```python
from build123d import *

# Parameters (mm, degrees)
F1_DEPTH = 10


with BuildPart() as f1:
    # F0 (on Front) → F1 (new body)
    with BuildSketch(Plane.XZ):
        with BuildLine():
            ThreePointArc((-34.337593, 36.377659), (-39.128216, 31.167084), (-43.135461, 25.332518))
            ThreePointArc((-43.135461, 25.332518), (-45.923647, 19.834894), (-48.014505, 14.036086))
            ThreePointArc((-48.014505, 14.036086), (-49.519107, 7.089604), (-50.024038, 0))
            ThreePointArc((-50.024038, 0), (-50.020463, -0.5981), (-50.009736, -1.196115))
            ThreePointArc((-50.009736, -1.196115), (-49.341893, -8.232983), (-47.688879, -15.105469))
            ThreePointArc((-47.688879, -15.105469), (-46.725007, -17.865557), (-45.601542, -20.564625))
            ThreePointArc((-45.601542, -20.564625), (-42.251133, -26.781453), (-38.058637, -32.464513))
            ThreePointArc((-38.058637, -32.464513), (-34.360112, -36.35639), (-30.265785, -39.82947))
            ThreePointArc((-30.265785, -39.82947), (-24.362413, -43.6907), (-17.974608, -46.683165))
            ThreePointArc((-17.974608, -46.683165), (-12.820651, -48.353235), (-7.516311, -49.456137))
            ThreePointArc((-7.516311, -49.456137), (-0.470356, -50.021827), (6.584991, -49.588732))
            ThreePointArc((6.584991, -49.588732), (11.499056, -48.684455), (16.298397, -47.294467))
            ThreePointArc((16.298397, -47.294467), (22.803128, -44.524395), (28.852373, -40.864961))
            ThreePointArc((28.852373, -40.864961), (32.363977, -38.144166), (35.620358, -35.122564))
            ThreePointArc((35.620358, -35.122564), (40.222649, -29.741266), (44.019019, -23.764057))
            ThreePointArc((44.019019, -23.764057), (45.828281, -20.054253), (47.32555, -16.207922))
            ThreePointArc((47.32555, -16.207922), (49.138207, -9.372354), (49.968834, -2.349478))
            ThreePointArc((49.968834, -2.349478), (50.010235, -1.175063), (50.024038, 0))
            ThreePointArc((50.024038, 0), (49.77315, 5.003793), (49.023002, 9.957394))
            ThreePointArc((49.023002, 9.957394), (47.119504, 16.797522), (44.266789, 23.299265))
            ThreePointArc((44.266789, 23.299265), (41.258147, 28.287272), (37.690051, 32.891708))
            ThreePointArc((37.690051, 32.891708), (32.67536, 37.877768), (27.007686, 42.10688))
            ThreePointArc((27.007686, 42.10688), (20.698662, 45.540858), (13.962862, 48.03585))
            ThreePointArc((13.962862, 48.03585), (7.051851, 49.524497), (0, 50.024038))
            ThreePointArc((0, 50.024038), (-7.417006, 49.471127), (-14.670053, 47.824616))
            ThreePointArc((-14.670053, 47.824616), (-21.285063, 45.269753), (-27.47235, 41.805196))
            ThreePointArc((-27.47235, 41.805196), (-31.023891, 39.241847), (-34.337593, 36.377659))
        make_face()
        with BuildLine():
            Line((-39.461789, 39.611867), (-43.135461, 25.332518))
            ThreePointArc((-43.135461, 25.332518), (-39.128216, 31.167084), (-34.337593, 36.377659))
            Line((-34.337593, 36.377659), (-39.461789, 39.611867))
        make_face()
        with BuildLine():
            ThreePointArc((-50.024038, 0), (-49.519107, 7.089604), (-48.014505, 14.036086))
            Line((-48.014505, 14.036086), (-54.538898, 14.036086))
            Line((-54.538898, 14.036086), (-50.024038, 0))
        make_face()
        with BuildLine():
            Line((-18.031633, 53.130766), (-27.47235, 41.805196))
            ThreePointArc((-27.47235, 41.805196), (-21.285063, 45.269753), (-14.670053, 47.824616))
            Line((-14.670053, 47.824616), (-18.031633, 53.130766))
        make_face()
        with BuildLine():
            ThreePointArc((-47.688879, -15.105469), (-49.341893, -8.232983), (-50.009736, -1.196115))
            Line((-50.009736, -1.196115), (-55.682706, -2.716183))
            Line((-55.682706, -2.716183), (-47.688879, -15.105469))
        make_face()
        with BuildLine():
            Line((14.219069, 53.924521), (0, 50.024038))
            ThreePointArc((0, 50.024038), (7.051851, 49.524497), (13.962862, 48.03585))
            Line((13.962862, 48.03585), (14.219069, 53.924521))
        make_face()
        with BuildLine():
            ThreePointArc((-38.058637, -32.464513), (-42.251133, -26.781453), (-45.601542, -20.564625))
            Line((-45.601542, -20.564625), (-50.161836, -24.043809))
            Line((-50.161836, -24.043809), (-38.058637, -32.464513))
        make_face()
        with BuildLine():
            Line((41.094992, 37.754468), (27.007686, 42.10688))
            ThreePointArc((27.007686, 42.10688), (32.67536, 37.877768), (37.690051, 32.891708))
            Line((37.690051, 32.891708), (41.094992, 37.754468))
        make_face()
        with BuildLine():
            ThreePointArc((-17.974608, -46.683165), (-24.362413, -43.6907), (-30.265785, -39.82947))
            Line((-30.265785, -39.82947), (-32.603685, -44.843111))
            Line((-32.603685, -44.843111), (-17.974608, -46.683165))
        make_face()
        with BuildLine():
            Line((54.722803, 12.903715), (44.266789, 23.299265))
            ThreePointArc((44.266789, 23.299265), (47.119504, 16.797522), (49.023002, 9.957394))
            Line((49.023002, 9.957394), (54.722803, 12.903715))
        make_face()
        with BuildLine():
            ThreePointArc((6.584991, -49.588732), (-0.470356, -50.021827), (-7.516311, -49.456137))
            Line((-7.516311, -49.456137), (-7.004188, -55.309737))
            Line((-7.004188, -55.309737), (6.584991, -49.588732))
        make_face()
        with BuildLine():
            ThreePointArc((28.852373, -40.864961), (22.803128, -44.524395), (16.298397, -47.294467))
            Line((16.298397, -47.294467), (19.493974, -52.258645))
            Line((19.493974, -52.258645), (28.852373, -40.864961))
        make_face()
        with BuildLine():
            Line((53.243188, -16.725649), (49.968834, -2.349478))
            ThreePointArc((49.968834, -2.349478), (49.138207, -9.372354), (47.32555, -16.207922))
            Line((47.32555, -16.207922), (53.243188, -16.725649))
        make_face()
        with BuildLine():
            ThreePointArc((44.019019, -23.764057), (40.222649, -29.741266), (35.620358, -35.122564))
            Line((35.620358, -35.122564), (40.910959, -38.177094))
            Line((40.910959, -38.177094), (44.019019, -23.764057))
        make_face()
    extrude(amount=F1_DEPTH)


solid = f1.part
```
Design review of the part built by this model. Coordinates are the model's own, in mm. A direction names the side the tool comes from. Give positions to 0.01 mm unless a question says otherwise; leave off trailing zeros. Loops run counter-clockwise (first coordinate to the right, second up) from the corner with the lowest first, then second, coordinate; pieces in that order, holes last. Notation, with made-up numbers: (58, 0.25) -> (72, 0.25) arc R35 ccw to (72, 38.25) -> close; hole circle Ø9 at (-2, 23.25). An arc over 180 degrees is marked (long way). One line per item, written item: value.
Q1. For pin 1 Ø6 at (x, y) = (27, -6.5) entering from +Z; pin 2 Ø3 at (y, z) = (-5.5, 28.5) entering from -X; pin 3 Ø5 at (y, z) = (-1, -3) entering from +X, all flat-tipped, find the tip position at first contact; note any pin that passes through.
Numbers:
pin 1: stops at z = 43.89
pin 2: stops at x = -42.71
pin 3: stops at x = 50.69
Q2. We need section A-A on z = 5. Give the boundary of the cut face in (x, y), and give its area (3 significant figures).
Numbers:
outline: (-51.63, -10) -> (49.77, -10) -> (49.77, 0) -> (-51.63, 0) -> close
area: 1,010 mm^2
Q3. We need section B-B on x = -4.5. Give the boundary of the cut face in (y, z), and give its area (3 significant figures).
Numbers:
outline: (-10, -54.26) -> (0, -54.26) -> (0, 49.82) -> (-10, 49.82) -> close
area: 1,040 mm^2
Q4. Machinability: for faces 5 (the flat face through (-51, -5, 14.036)), 6 (the cylindrical face through (41.304, -4.93, 28.22)), 7 (the flat face through (-36.86, -4.93, 37.97)), 8 (the flat face through (-31.42, -4.93, -42.3)), which of the approach directions +Z, -Z, +X, -X, +Y, -Y give a long, thin tool a straight path to every point of the face, cutting with its end or side? Answer none if there is none.
Numbers:
face 5: +Z, -X, +Y, -Y
face 6: +X, +Y, -Y
face 7: +Z, +Y, -Y
face 8: -X, +Y, -Y
Q5. For L1, parallel to Z at x = 44.5, y = -5.5; L2, parallel to X at y = -1.75, z = 46; L3, parallel to Z at x = -2, y = -4.75, list the stretches that pass through material, from the lowest coordinate up.
Numbers:
L1: z = -22.85 to 23.07
L2: x = -23.98 to 19.66
L3: z = -53.2 to 49.98
Q6. Draft analysis for pull direction X (two halves, no side actions). For faces 1 (the flat face through (-1, 0, 0)), 2 (the flat face through (17.874, -4.93, -49.742)), 3 (the flat face through (-44.19, -4.93, -28.2)), 4 (the cylindrical face through (-30.976, -4.93, 39.28)), state which applies: pulls with the +X half, pulls with the -X half, needs draft (parallel to the pull), parting line crosses it, or undercut.
Numbers:
face 1: needs draft
face 2: undercut
face 3: pulls with the -X half
face 4: undercut
